from build123d import *

# Parameters (mm, degrees)
SKETCH1_R           = 26
SKETCH1_R_2         = 1.5
SKETCH1_R_3         = 4.5
BOSS_EXTRUDE1_DEPTH = 2
SKETCH1_2_R         = 4.5
BOSS_EXTRUDE2_DEPTH = 4.5
SKETCH2_R           = 1.5
CUT_EXTRUDE1_DEPTH  = 4.5
SKETCH3_R           = 2.75
CUT_EXTRUDE2_DEPTH  = 3.5
CUT_EXTRUDE3_DEPTH  = 3.5
CIRPATTERN1_COUNT   = 25
SKETCH5_R           = 18.5
SKETCH5_R_2         = 1.5
BOSS_EXTRUDE3_DEPTH = 3


with BuildPart() as part:
    # Sketch1 → Boss-Extrude1 (new body)
    with BuildSketch(Plane.XY):
        Circle(SKETCH1_R)
        with Locations((0, 22)):
            Circle(SKETCH1_R_2, mode=Mode.SUBTRACT)
        with Locations((22, 0)):
            Circle(SKETCH1_R_2, mode=Mode.SUBTRACT)
        with Locations((0, -22)):
            Circle(SKETCH1_R_2, mode=Mode.SUBTRACT)
        with Locations((-22, 0)):
            Circle(SKETCH1_R_2, mode=Mode.SUBTRACT)
        Circle(SKETCH1_R_3, mode=Mode.SUBTRACT)
    extrude(amount=BOSS_EXTRUDE1_DEPTH)

    # Sketch1_2 → Boss-Extrude2 (add)
    with BuildSketch(Plane.XY):
        Circle(SKETCH1_2_R)
    extrude(amount=BOSS_EXTRUDE2_DEPTH)

    # Sketch2 → Cut-Extrude1 (cut)
    with BuildSketch(Plane(origin=(0, 0, 0), x_dir=(-1, 0, 0), z_dir=(0, 0, -1))):
        Circle(SKETCH2_R)
    extrude(amount=-CUT_EXTRUDE1_DEPTH, mode=Mode.SUBTRACT)

    # Sketch3 → Cut-Extrude2 (cut)
    with BuildSketch(Plane.XY.offset(4.5)):
        Circle(SKETCH3_R)
    extrude(amount=-CUT_EXTRUDE2_DEPTH, mode=Mode.SUBTRACT)

    # Sketch4 → Cut-Extrude3 (cut)
    with BuildSketch(Plane.XY.offset(4.5)):
        with BuildLine():
            Line((-2.976344104, 0.375999701), (-2.728315429, 0.344666392))
            ThreePointArc((-2.728315429, 0.344666392), (-2.70218519, 0.510583192), (-2.665974712, 0.674595311))
            Line((-2.665974712, 0.674595311), (-2.976344104, 0.375999701))
        make_face()
        with BuildLine():
            Line((-2.976344104, 0.375999701), (-2.75, 0))
            ThreePointArc((-2.75, 0), (-2.744573503, 0.172673929), (-2.728315429, 0.344666392))
            Line((-2.728315429, 0.344666392), (-2.976344104, 0.375999701))
        make_face()
    cut_extrude3 = extrude(amount=-CUT_EXTRUDE3_DEPTH, mode=Mode.SUBTRACT)

    # CirPattern1: Cut-Extrude3 ×25 about axis
    cirpattern1_axis = Axis((0, 0, 0), (0, 0, 1))
    for i in range(1, CIRPATTERN1_COUNT):
        add(cut_extrude3.rotate(cirpattern1_axis, i * 360 / CIRPATTERN1_COUNT), mode=Mode.SUBTRACT)

    # Sketch5 → Boss-Extrude3 (add)
    with BuildSketch(Plane(origin=(0, 0, 0), x_dir=(-1, 0, 0), z_dir=(0, 0, -1))):
        Circle(SKETCH5_R)
        Circle(SKETCH5_R_2, mode=Mode.SUBTRACT)
    extrude(amount=BOSS_EXTRUDE3_DEPTH)


solid = part.part
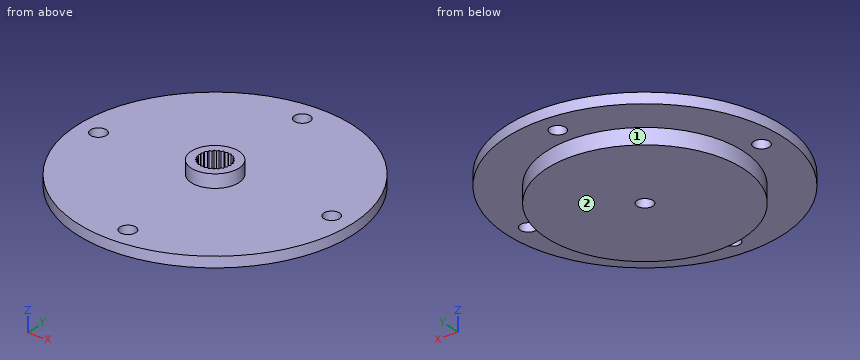
For this review, take the finished solid that the model builds, in its own axes (mm). Face numbers are marked on the shaded views. A direction names the side the tool comes from. Round coordinates to 2 decimals unless told otherwise and drop trailing zeros. Order: outer loops, then holes, each group sorted by start corner. A loop starts at its lowest first (then second) coordinate and runs counter-clockwise, first axis right, second up. Notation, with made-up numbers: M 86,81 L 95,81 A24 ccw 95,100 Z; hole C -2,-7 d7. An arc over 180 degrees is marked long. Use a Markdown table: item, result. Add a question column.
Item 1: Add section A-A, the plane y = 22. Give the boundary of the cut face in (x, z).
Item 2: Add section D-D, the plane y = 6. Give the boundary of the cut face in (x, z).
Item 3: Add section C-C, the plane z = -1.5. Give the boundary of the cut face in (x, y).
Item 4: Insertion check: pin 1 (5 mm diameter, centred on x = 0, y = -22, fed in from +Z); pin 2 (1 mm diameter, centred on y = 17, z = 2, fed in from +X); pin 3 (2.5 mm diameter, centred on x = 0, y = 0, fed in from -Z); pin 4 (4 mm diameter, centred on x = 0, y = 0, fed in from +Z). Each pin has a flat end and moves straight along its axis. Give the tip position at first contact, or say it passes through.
Item 5: To check wall thickness, follow line 1 along Y through (x, z) = (0, 1.55); line 2 along Y through (x, z) = (0, 3.75); line 3 along Z through (x, y) = (-7.5, -20). State the ranges of each line that lie inside material, in increasing order.
Item 6: Tool access review of the marked faces 1 and 2: name each direction out of +Z, -Z, +X, -X, +Y, -Y from which nothing blocks a thin tool from reaching the whole face with its end or side.
Geometry results:
| question | item | result |
|---|---|---|
| 1 | outline | M -13.86,0 L -1.5,0 L -1.5,2 L -13.86,2 Z; M 1.5,0 L 13.86,0 L 13.86,2 L 1.5,2 Z |
| 2 | outline | M -25.3,0 L -17.5,0 L -17.5,-3 L 17.5,-3 L 17.5,0 L 25.3,0 L 25.3,2 L -25.3,2 Z |
| 3 | outline | C 0,0 d37; hole C 0,0 d3 |
| 4 | pin 1 | stops at z = 2 |
| 4 | pin 2 | stops at x = 20.09 |
| 4 | pin 3 | passes through |
| 4 | pin 4 | stops at z = 1 |
| 5 | line 1 | y = -26 to -23.5, -20.5 to -2.86, 2.86 to 20.5, 23.5 to 26 |
| 5 | line 2 | y = -4.5 to -2.86, 2.86 to 4.5 |
| 5 | line 3 | z = 0 to 2 |
| 6 | face 1 | -Z |
| 6 | face 2 | -Z, +X, -X, +Y, -Y |
